Could you check a few things on this model? Use its own coordinates, in mm. A direction names the side the tool comes from. Round coordinates to 2 decimals unless told otherwise and drop trailing zeros. Order: outer loops, then holes, each group sorted by start corner. A loop starts at its lowest first (then second) coordinate and runs counter-clockwise, first axis right, second up. Notation, with made-up numbers: (45.25, 57.25) - (96.25, 57.25) arc R7 cw to (96.25, 64.25) - close; hole circle Ø5 at (52.25, 74.5). An arc over 180 degrees is marked (long way). Use one line per item in the form item = value.
from build123d import *

# Parameters (mm, degrees)
EXTRUDE_1_DEPTH          = 1
EXTRUDE_START            = 5
EXTRUDE_2_DEPTH          = 5
CUT_EXTRUDE_2_DEPTH      = 5
EXTRUDE_3_DEPTH          = 3.4
CUT_EXTRUDE_3_DEPTH      = 94.28451104
CUT_EXTRUDE_3_DEPTH_BACK = 94.28451104
SKETCH_4_R               = 1
SKETCH_7_R               = 1
CUT_EXTRUDE_8_DEPTH      = 94.28451104
SKETCH_8_R               = 2.6
CUT_EXTRUDE_9_DEPTH      = 2
SKETCH_9_W               = 1
SKETCH_9_H               = 26
EXTRUDE_4_DEPTH          = 5.2
CUT_EXTRUDE_11_REACH     = 96.573
SKETCH_10_R              = 2
SKETCH_10_W              = 2
SKETCH_10_H              = 4


with BuildPart() as part:
    # Sketch 1 → Extrude 1 (new body)
    with BuildSketch(Plane(origin=(0, 0, 0), x_dir=(1, 0, 0), z_dir=(0, 1, 0))):
        with BuildLine():
            Line((3, -1), (77, -1))
            ThreePointArc((77, -1), (79.828427125, 0.171572875), (81, 3))
            Line((81, 3), (81, 42))
            ThreePointArc((81, 42), (79.828427125, 44.828427125), (77, 46))
            Line((77, 46), (3, 46))
            ThreePointArc((3, 46), (0.171572875, 44.828427125), (-1, 42))
            Line((-1, 42), (-1, 3))
            ThreePointArc((-1, 3), (0.171572875, 0.171572875), (3, -1))
        make_face()
    extrude(amount=-EXTRUDE_1_DEPTH)

    # Sketch 1_3 → Extrude 2 (add)
    with BuildSketch(Plane(origin=(0, 0, 0), x_dir=(1, 0, 0), z_dir=(0, 1, 0)).offset(EXTRUDE_START)):
        with BuildLine():
            Line((3, -1), (77, -1))
            ThreePointArc((77, -1), (79.828427125, 0.171572875), (81, 3))
            Line((81, 3), (81, 42))
            ThreePointArc((81, 42), (79.828427125, 44.828427125), (77, 46))
            Line((77, 46), (3, 46))
            ThreePointArc((3, 46), (0.171572875, 44.828427125), (-1, 42))
            Line((-1, 42), (-1, 3))
            ThreePointArc((-1, 3), (0.171572875, 0.171572875), (3, -1))
        make_face()
    extrude(amount=-EXTRUDE_2_DEPTH)

    # Sketch 6 → Cut-Extrude 2 (cut)
    with BuildSketch(Plane(origin=(0, 0, 0), x_dir=(1, 0, 0), z_dir=(0, 1, 0))):
        with BuildLine():
            Line((80, 3), (80, 42))
            ThreePointArc((80, 42), (79.121320344, 44.121320344), (77, 45))
            Line((77, 45), (3, 45))
            ThreePointArc((3, 45), (0.878679656, 44.121320344), (0, 42))
            Line((0, 42), (0, 3))
            ThreePointArc((0, 3), (0.878679656, 0.878679656), (3, 0))
            Line((3, 0), (77, 0))
            ThreePointArc((77, 0), (79.121320344, 0.878679656), (80, 3))
        make_face()
    extrude(amount=CUT_EXTRUDE_2_DEPTH, mode=Mode.SUBTRACT)

    # Sketch 5 → Extrude 3 (add)
    with BuildSketch(Plane(origin=(0, 0, 0), x_dir=(1, 0, 0), z_dir=(0, 1, 0))):
        with BuildLine():
            Line((77, 6), (80, 6))
            Line((80, 6), (80, 3))
            ThreePointArc((80, 3), (79.121320344, 0.878679656), (77, 0))
            Line((77, 0), (74, 0))
            Line((74, 0), (74, 3))
            ThreePointArc((74, 3), (74.878679656, 5.121320344), (77, 6))
        make_face()
        with BuildLine():
            Line((77, 45), (74, 45))
            Line((74, 45), (74, 42))
            ThreePointArc((74, 42), (74.878679656, 39.878679656), (77, 39))
            Line((77, 39), (80, 39))
            Line((80, 39), (80, 42))
            ThreePointArc((80, 42), (79.121320344, 44.121320344), (77, 45))
        make_face()
        with BuildLine():
            Line((0, 42), (0, 39))
            Line((0, 39), (3, 39))
            ThreePointArc((3, 39), (5.121320344, 39.878679656), (6, 42))
            Line((6, 42), (6, 45))
            Line((6, 45), (3, 45))
            ThreePointArc((3, 45), (0.878679656, 44.121320344), (0, 42))
        make_face()
        with BuildLine():
            Line((3, 6), (0, 6))
            Line((0, 6), (0, 3))
            ThreePointArc((0, 3), (0.878679656, 0.878679656), (3, 0))
            Line((3, 0), (6, 0))
            Line((6, 0), (6, 3))
            ThreePointArc((6, 3), (5.121320344, 5.121320344), (3, 6))
        make_face()
    extrude(amount=EXTRUDE_3_DEPTH)

    # Sketch 4 → Cut-Extrude 3 (cut, two sides: drawn at the far end of the back side and taken through both)
    with BuildSketch(Plane(origin=(0, 0, 0), x_dir=(1, 0, 0), z_dir=(0, 1, 0)).offset(-CUT_EXTRUDE_3_DEPTH_BACK)):
        with Locations(Location((3, 42, 0), (0, 0, 270))):
            Circle(SKETCH_4_R)
        with Locations(Location((3, 3, 0), (0, 0, 270))):
            Circle(SKETCH_4_R)
        with Locations(Location((77, 3, 0), (0, 0, 270))):
            Circle(SKETCH_4_R)
        with Locations(Location((77, 42, 0), (0, 0, 270))):
            Circle(SKETCH_4_R)
    extrude(amount=CUT_EXTRUDE_3_DEPTH + CUT_EXTRUDE_3_DEPTH_BACK, mode=Mode.SUBTRACT)

    # Sketch 7 → Cut-Extrude 8 (cut, through all)
    with BuildSketch(Plane(origin=(0, 0, 0), x_dir=(1, 0, 0), z_dir=(0, 1, 0))):
        with Locations(Location((50.3, 13.3, 0), (0, 0, 270))):
            Circle(SKETCH_7_R)
        with Locations(Location((57.8, 38.3, 0), (0, 0, 270))):
            Circle(SKETCH_7_R)
    extrude(amount=-CUT_EXTRUDE_8_DEPTH, mode=Mode.SUBTRACT)

    # Sketch 8 → Cut-Extrude 9 (cut)
    with BuildSketch(Plane.XZ.offset(1)):
        with Locations(Location((3, -3, 0), (0, 0, 270))):
            Circle(SKETCH_8_R)
        with Locations(Location((77, -3, 0), (0, 0, 270))):
            Circle(SKETCH_8_R)
        with Locations(Location((3, -42, 0), (0, 0, 270))):
            Circle(SKETCH_8_R)
        with Locations(Location((77, -42, 0), (0, 0, 270))):
            Circle(SKETCH_8_R)
    extrude(amount=-CUT_EXTRUDE_9_DEPTH, mode=Mode.SUBTRACT)

    # Sketch 9 → Extrude 4 (add)
    with BuildSketch(Plane(origin=(0, 5, 0), x_dir=(1, 0, 0), z_dir=(0, 1, 0))):
        with Locations((80.5, 22.5)):
            Rectangle(SKETCH_9_W, SKETCH_9_H)
    extrude(amount=EXTRUDE_4_DEPTH)

    # Sketch 10 → Cut-Extrude 11 (cut, up to next)
    with BuildSketch(Plane(origin=(81, 0, 0), x_dir=(0, 0, -1), z_dir=(1, 0, 0)), mode=Mode.PRIVATE) as cut_extrude_11_sk1:
        with Locations((22.5, 10.2)):
            Circle(SKETCH_10_R)
    cut_extrude_11_tool1 = extrude(cut_extrude_11_sk1.sketch, amount=-CUT_EXTRUDE_11_REACH, mode=Mode.PRIVATE) & part.part
    # Sketch 10 → Cut-Extrude 11 (cut, up to next)
    with BuildSketch(Plane(origin=(81, 0, 0), x_dir=(0, 0, -1), z_dir=(1, 0, 0)), mode=Mode.PRIVATE) as cut_extrude_11_sk2:
        with Locations((10.5, 10.2)):
            Rectangle(SKETCH_10_W, SKETCH_10_H)
    cut_extrude_11_tool2 = extrude(cut_extrude_11_sk2.sketch, amount=-CUT_EXTRUDE_11_REACH, mode=Mode.PRIVATE) & part.part
    # Sketch 10 → Cut-Extrude 11 (cut, up to next)
    with BuildSketch(Plane(origin=(81, 0, 0), x_dir=(0, 0, -1), z_dir=(1, 0, 0)), mode=Mode.PRIVATE) as cut_extrude_11_sk3:
        with Locations((34.5, 10.2)):
            Rectangle(SKETCH_10_W, SKETCH_10_H)
    cut_extrude_11_tool3 = extrude(cut_extrude_11_sk3.sketch, amount=-CUT_EXTRUDE_11_REACH, mode=Mode.PRIVATE) & part.part
    add(cut_extrude_11_tool1.solids().sort_by_distance((81, 10.2, -22.5))[0], mode=Mode.SUBTRACT)
    add(cut_extrude_11_tool2.solids().sort_by_distance((81, 10.2, -10.5))[0], mode=Mode.SUBTRACT)
    add(cut_extrude_11_tool3.solids().sort_by_distance((81, 10.2, -34.5))[0], mode=Mode.SUBTRACT)


solid = part.part
Item 1: Imagine slicing it at C-C on y = 2. Please give me the cut outline in (x, z), plus the area to 3 significant figures.
Found:
outline = (-1, -42) arc R4 ccw to (3, -46) - (77, -46) arc R4 ccw to (81, -42) - (81, -3) arc R4 ccw to (77, 1) - (3, 1) arc R4 ccw to (-1, -3) - close; hole (0, -39) - (3, -39) arc R3 cw to (6, -42) - (6, -45) - (74, -45) - (74, -42) arc R3 cw to (77, -39) - (80, -39) - (80, -6) - (77, -6) arc R3 cw to (74, -3) - (74, 0) - (6, 0) - (6, -3) arc R3 cw to (3, -6) - (0, -6) - close; hole circle Ø2 at (3, -42); hole circle Ø2 at (3, -3); hole circle Ø2 at (77, -42); hole circle Ø2 at (77, -3)
area = 364 mm2
Item 2: Will these pins go through, and if not, where does the flat tip stop? P1, Ø2.5, axis at x = 3, z = -3, coming from the -Y side; P2, Ø10, axis at x = 32.5, z = -13.5, coming from the +Y side; P3, Ø5, axis at x = 2, z = -42, coming from the +Y side.
Found:
P1 = 1
P2 = 0
P3 = 5
Item 3: Imagine slicing it at A-A on z = -13.3. Please give me the cut outline in (x, y), plus the area to 3 significant figures.
Found:
outline = (-1, -1) - (49.3, -1) - (49.3, 0) - (0, 0) - (0, 5) - (-1, 5) - close; (51.3, -1) - (81, -1) - (81, 10.2) - (80, 10.2) - (80, 0) - (51.3, 0) - close
area = 95.2 mm2
Item 4: If we mould it in two halves opening along Z, with no side actions, what happens to faces 1 (the face through (-1, 2, -23)), 2 (the face through (41, 2, -45))? For each: released by +Z, released by -Z, zero draft, split by the parting line, or undercut.
Found:
face_1 = zero draft
face_2 = undercut
Item 5: Imagine slicing it at B-B on x = 57.8. Please give me the cut outline in (y, z), plus the area to 3 significant figures.
Found:
outline = (-1, -46) - (5, -46) - (5, -45) - (0, -45) - (0, -39.3) - (-1, -39.3) - close; (-1, -37.3) - (0, -37.3) - (0, 0) - (5, 0) - (5, 1) - (-1, 1) - close
area = 55.0 mm2
Item 6: I need wall thicknesses on L1, parallel to Z at x = 77, y = 2.45; L2, parallel to X at y = 0.4, z = -42; L3, parallel to X at y = 2.45, z = -42. Which ranges of each line are inside material? Lowest first, please.
Found:
L1 = -46 to -43, -41 to -39, -6 to -4, -2 to 1
L2 = -1 to 0.4, 5.6 to 6, 74 to 74.4, 79.6 to 81
L3 = -1 to 2, 4 to 6, 74 to 76, 78 to 81
Item 7: Imagine slicing it at D-D on x = 40. Please give me the cut outline in (y, z).
Found:
outline = (-1, -46) - (5, -46) - (5, -45) - (0, -45) - (0, 0) - (5, 0) - (5, 1) - (-1, 1) - close
Item 8: For faces 3 (the face through (5.14, 1.68, -5.1)), 4 (the face through (49.324, -0.493, -13.517)), 5 (the face through (1.418, -0.014, -0.937)), which set-ups out of +Z, -Z, +X, -X, +Y, -Y let a thin tool reach every point of the face, with its end or its side?
Found:
face_3 = +Y
face_4 = +Y, -Y
face_5 = -Y
